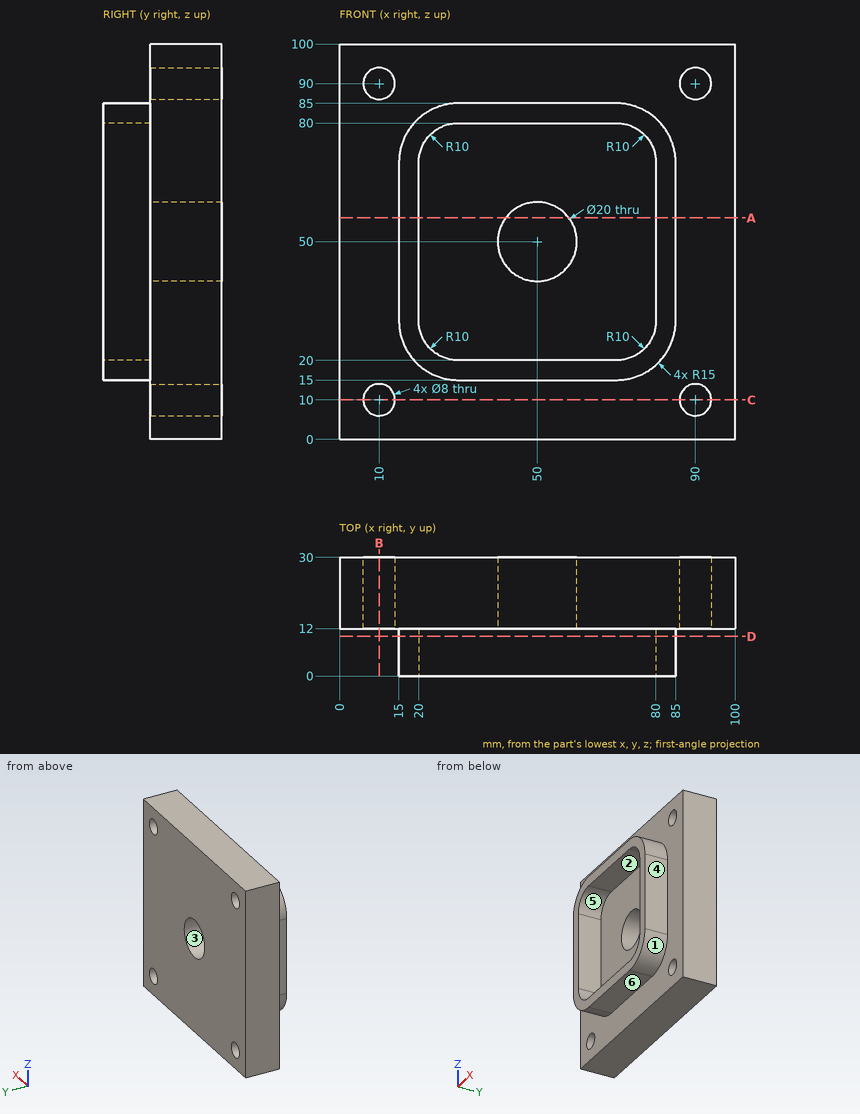
Part print with two shaded views. Sizes in mm from the minimum x, y, z corner. A direction names the side the tool comes from. Round coordinates to 2 decimals unless told otherwise and drop trailing zeros. Loops run counter-clockwise (first coordinate to the right, second up) from the corner with the lowest first, then second, coordinate; pieces in that order, holes last. Notation, with made-up numbers: (-0.75, 26) - (31.25, 26) arc R4 cw to (31.25, 30) - close; hole circle Ø1 at (-30, 8). An arc over 180 degrees is marked (long way). Put each result on its own line as item: value.
1. Slice it at D-D on y = 10. List the corners of the cut face in (x, z), and give its area (3 significant figures).
Geometry check:
outline: (15, 30) arc R15 ccw to (30, 15) - (70, 15) arc R15 ccw to (85, 30) - (85, 70) arc R15 ccw to (70, 85) - (30, 85) arc R15 ccw to (15, 70) - close; hole (20, 30) arc R10 ccw to (30, 20) - (70, 20) arc R10 ccw to (80, 30) - (80, 70) arc R10 ccw to (70, 80) - (30, 80) arc R10 ccw to (20, 70) - close
area: 1,190 mm²
2. Slice it at B-B on x = 10. List the corners of the cut face in (y, z), and give its area (3 significant figures).
Geometry check:
outline: (12, 0) - (30, 0) - (30, 6) - (12, 6) - close; (12, 14) - (30, 14) - (30, 86) - (12, 86) - close; (12, 94) - (30, 94) - (30, 100) - (12, 100) - close
area: 1,510 mm²
3. Wall check: line 1 (Z direction, x = 90, y = 24); line 2 (Z direction, x = 50, y = 18.25); line 3 (X direction, y = 5.75, z = 65). Give the ranges that are in metal, low to high.
Geometry check:
line 1: 0 to 6, 14 to 86, 94 to 100
line 2: 0 to 40, 60 to 100
line 3: 15 to 20, 80 to 85
4. Two-plate mould, pull along X, no slides. Class the marked faces 4, 5 and 6: released by +X, released by -X, zero draft, split by the parting line, or undercut.
Geometry check:
face 4: released by +X
face 5: undercut
face 6: zero draft
5. Slice it at C-C on z = 10. List the corners of the cut face in (x, y), and give its area (3 significant figures).
Geometry check:
outline: (0, 12) - (6, 12) - (6, 30) - (0, 30) - close; (14, 12) - (86, 12) - (86, 30) - (14, 30) - close; (94, 12) - (100, 12) - (100, 30) - (94, 30) - close
area: 1,510 mm²
6. Slice it at A-A on z = 56. List the corners of the cut face in (x, y), and give its area (3 significant figures).
Geometry check:
outline: (0, 12) - (15, 12) - (15, 0) - (20, 0) - (20, 12) - (42, 12) - (42, 30) - (0, 30) - close; (58, 12) - (80, 12) - (80, 0) - (85, 0) - (85, 12) - (100, 12) - (100, 30) - (58, 30) - close
area: 1,630 mm²
7. 3-axis set-ups, long thin cutter, end or side, ignore diameter. For the marked faces 1, 2 and 3: which of +Z, -Z, +X, -X, +Y, -Y reach the whole face in a straight line?
Geometry check:
face 1: -Z, +X, -Y
face 2: -Y
face 3: +Y, -Y
8. Pin check, flat tips, straight feed: P1, Ø6, axis at y = 6.5, z = 44, coming from the -X side; P2, Ø9, axis at x = 90, z = 10, coming from the -Y side; P3, Ø3.5, axis at x = 58.5, y = 8, coming from the +Z side. Stop position of each tip, or through.
Geometry check:
P1: x = 15
P2: y = 12
P3: z = 85
